Print and shaded views of the part. All mm, measured from the part's lowest x, y and z. A direction names the side the tool comes from. Give positions to 0.01 mm unless a question says otherwise; leave off trailing zeros. Order: outer loops, then holes, each group sorted by start corner. A loop starts at its lowest first (then second) coordinate and runs counter-clockwise, first axis right, second up. Notation, with made-up numbers: (70, 16) - (77, 16) arc R24 ccw to (77, 38) - close; hole circle Ø3 at (15.5, 88). An arc over 180 degrees is marked (long way). Answer in a Markdown table with one row per item.
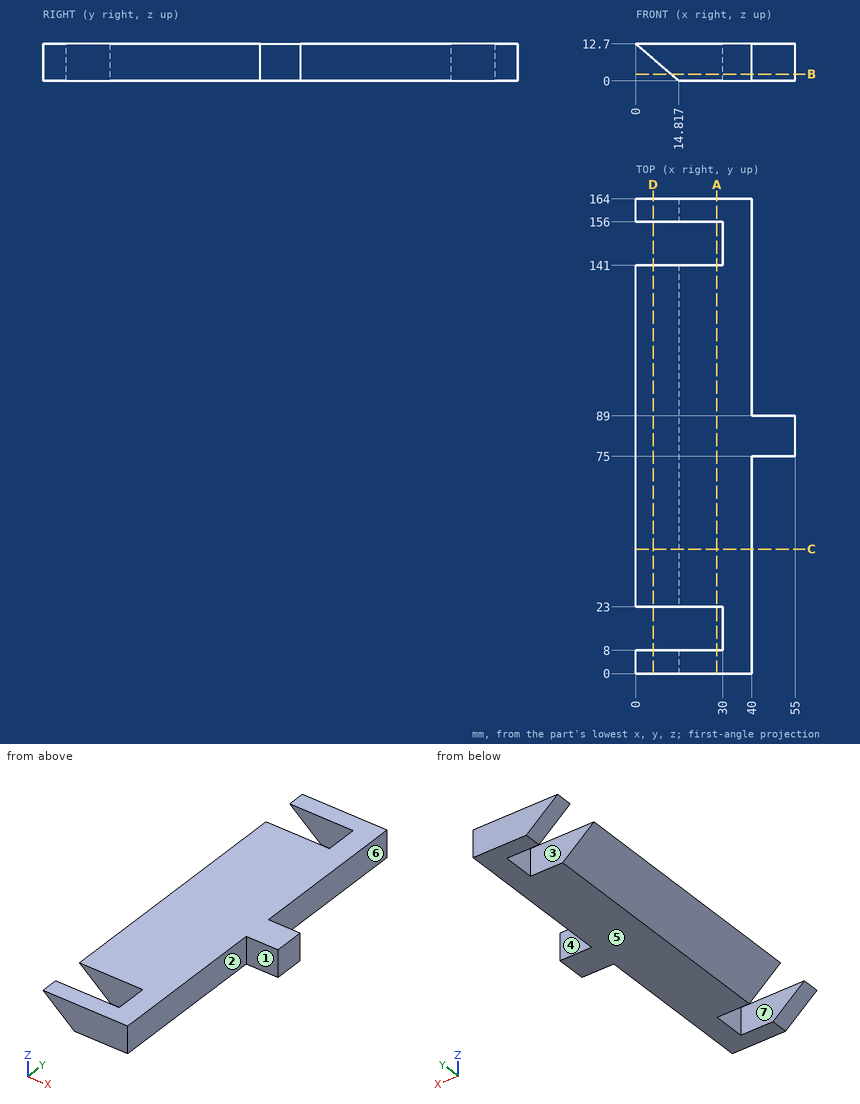
1. Cut at B-B on z = 2.25. Write the cut outline in (x, y).
Check result:
| item | result |
|---|---|
| outline | (12.19, 0) - (40, 0) - (40, 75) - (55, 75) - (55, 89) - (40, 89) - (40, 164) - (12.19, 164) - (12.19, 156) - (30, 156) - (30, 141) - (12.19, 141) - (12.19, 23) - (30, 23) - (30, 8) - (12.19, 8) - close |
2. Cut at A-A on x = 28. Write the cut outline in (y, z), and give its area (3 significant figures).
Check result:
| item | result |
|---|---|
| outline | (0, 0) - (8, 0) - (8, 12.7) - (0, 12.7) - close; (23, 0) - (141, 0) - (141, 12.7) - (23, 12.7) - close; (156, 0) - (164, 0) - (164, 12.7) - (156, 12.7) - close |
| area | 1,700 mm² |
3. Cut at C-C on y = 43. Write the cut outline in (x, z), and give its area (3 significant figures).
Check result:
| item | result |
|---|---|
| outline | (0, 12.7) - (14.82, 0) - (40, 0) - (40, 12.7) - close |
| area | 414 mm² |
4. Two-plate mould, pull along Y, no slides. Class the marked faces 1, 2, 3 and 4: +Y half, -Y half, draft (parallel to the pull), parting line (faces both ways), or undercut.
Check result:
| item | result |
|---|---|
| face 1 | -Y half |
| face 2 | draft |
| face 3 | undercut |
| face 4 | +Y half |
5. Probe line 1 (Y direction, x = 28, z = 12.25); line 2 (X direction, y = 155.5, z = 4.5); line 3 (Y direction, x = 52, z = 6.25). List the from-to ranges inside material, lowest first.
Check result:
| item | result |
|---|---|
| line 1 | y = 0 to 8, 23 to 141, 156 to 164 |
| line 2 | x = 30 to 40 |
| line 3 | y = 75 to 89 |
6. Drop flat-ended pins along their axis: P1, Ø2, axis at y = 84, z = 1.5, coming from the -X side; P2, Ø4, axis at x = 49, z = 7.5, coming from the -Y side; P3, Ø5, axis at y = 130, z = 8, coming from the -X side. Give the stop position or say it passes through.
Check result:
| item | result |
|---|---|
| P1 | stops at x = 11.9 |
| P2 | stops at y = 75 |
| P3 | stops at x = 2.57 |
7. Cut at D-D on x = 6. Write the cut outline in (y, z).
Check result:
| item | result |
|---|---|
| outline | (0, 7.56) - (8, 7.56) - (8, 12.7) - (0, 12.7) - close; (23, 7.56) - (141, 7.56) - (141, 12.7) - (23, 12.7) - close; (156, 7.56) - (164, 7.56) - (164, 12.7) - (156, 12.7) - close |
8. Which spindle directions (+Z, -Z, +X, -X, +Y, -Y) get a long thin tool onto all of the face, cutting with end or side? Do the marked faces 5, 6 and 7. Say none if no direction does.
Check result:
| item | result |
|---|---|
| face 5 | -Z, +X, -X, +Y, -Y |
| face 6 | +Z, -Z, +X, +Y |
| face 7 | +Z, -Z, -X |
